Drawing for the job (mm, zero at the part's lowest x, y, z). A direction names the side the tool comes from. Give positions to 0.01 mm unless a question says otherwise; leave off trailing zeros. Order: outer loops, then holes, each group sorted by start corner. A loop starts at its lowest first (then second) coordinate and runs counter-clockwise, first axis right, second up. Notation, with made-up numbers: (62, 48.25) -> (83, 48.25) arc R28 ccw to (83, 69.25) -> close; hole circle Ø5 at (65.5, 76). An arc over 180 degrees is marked (long way). One line per item, written item: value. Start each with the question number.
(1) Saw through at C-C on x = 24. Give the cut face in (y, z).
(2) Saw through at B-B on z = 20. Give the cut face in (x, y), plus the area to 3 significant figures.
(3) Pin check, flat tips, straight feed: pin 1 (1.9 mm diameter, centred on y = 21.5, z = 30.5, fed in from -X); pin 2 (1.9 mm diameter, centred on x = 20, y = 4.5, fed in from +Z); pin 3 (2 mm diameter, centred on x = 26, z = 17, fed in from -Y). Stop position of each tip, or through.
(4) Saw through at A-A on y = 23.25. Give the cut face in (x, z).
(5) Which spindle directions (+Z, -Z, +X, -X, +Y, -Y) get a long thin tool onto all of the face, cutting with end or side? Do the marked faces 1, 2 and 3. Say none if no direction does.
(6) Saw through at D-D on y = 11. Give the cut face in (x, z).
(7) Probe line 1 (Y direction, x = 33.5, z = 30); line 2 (X direction, y = 20.25, z = 23); line 3 (Z direction, x = 6, y = 3.5). List the from-to ranges inside material, lowest first.
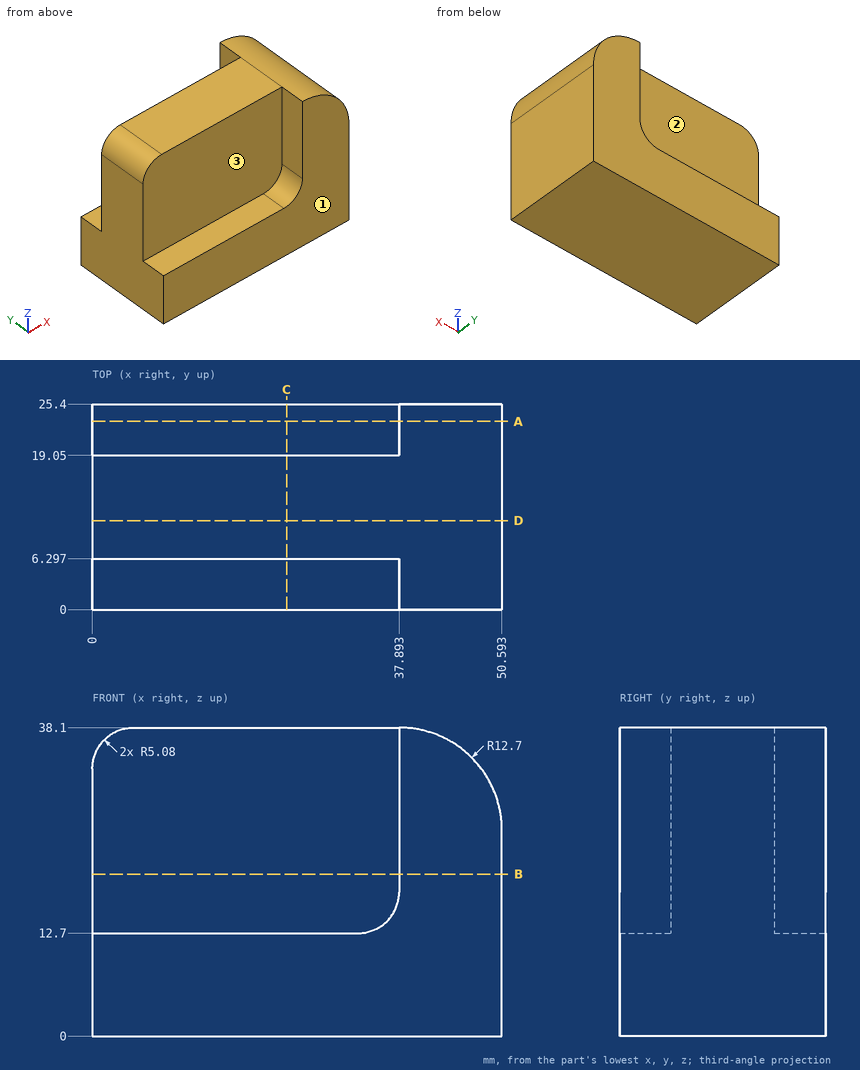
Results below:
1. outline: (0, 0) -> (25.4, 0) -> (25.4, 12.7) -> (19.05, 12.7) -> (19.05, 38.1) -> (6.3, 38.1) -> (6.3, 12.7) -> (0, 12.7) -> close
2. outline: (0, 6.3) -> (37.89, 6.3) -> (37.89, 0) -> (50.59, 0) -> (50.59, 25.4) -> (37.89, 25.4) -> (37.89, 19.05) -> (0, 19.05) -> close
2. area: 806 mm²
3. pin 1: stops at x = 37.89
3. pin 2: stops at z = 12.7
3. pin 3: stops at y = 6.3
4. outline: (0, 0) -> (50.59, 0) -> (50.59, 25.4) arc R12.7 ccw to (37.89, 38.1) -> (37.89, 17.78) arc R5.08 cw to (32.81, 12.7) -> (0, 12.7) -> close
5. face 1: +Z, -Z, +X, -X, -Y
5. face 2: +Z, -X, +Y
5. face 3: +Z, -X, -Y
6. outline: (0, 0) -> (50.59, 0) -> (50.59, 25.4) arc R12.7 ccw to (37.89, 38.1) -> (5.08, 38.1) arc R5.08 ccw to (0, 33.02) -> close
7. line 1: y = 6.3 to 19.05
7. line 2: x = 37.89 to 50.59
7. line 3: z = 0 to 12.7
